Part print with two shaded views. Sizes in mm from the minimum x, y, z corner. Coordinates: 2 decimals unless noted, no trailing zeros. Loops run counter-clockwise (first coordinate to the right, second up) from the corner with the lowest first, then second, coordinate; pieces in that order, holes last.
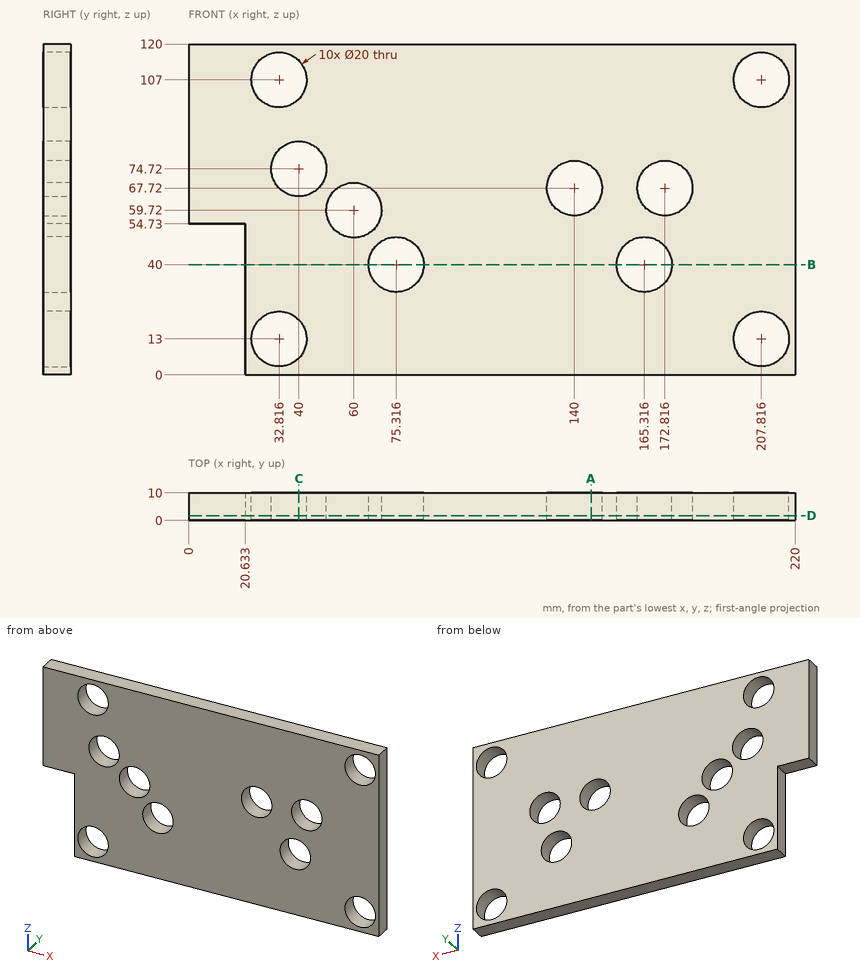
Q1. Drill centre lines: line 1 (X direction, y = 4.75, z = 13); line 2 (X direction, y = 5.5, z = 40); line 3 (X direction, y = 2.5, z = 67.72) (1 decimal). Where is each one in solid material? Low to high.
Answers:
line 1: x = 20.63 to 22.82, 42.82 to 197.82, 217.82 to 220
line 2: x = 20.63 to 65.32, 85.32 to 155.32, 175.32 to 220
line 3: x = 0 to 32.9, 47.1 to 54, 66 to 130, 150 to 162.8, 182.8 to 220
Q2. Flat gauge pins, fed straight in: P1, Ø23, axis at x = 207.82, z = 107, coming from the +Y side; P2, Ø5, axis at y = 3.5, z = 22.5, coming from the -X side. Where does each tip first touch, or does it go through?
Answers:
P1: stops at y = 10
P2: stops at x = 20.63
Q3. Slice it at C-C (x = 40). List the corners of the cut face in (y, z), and give its area (3 significant figures).
Answers:
outline: (0, 0) - (10, 0) - (10, 6.04) - (0, 6.04) - close; (0, 19.96) - (10, 19.96) - (10, 64.72) - (0, 64.72) - close; (0, 84.72) - (10, 84.72) - (10, 100.04) - (0, 100.04) - close; (0, 113.96) - (10, 113.96) - (10, 120) - (0, 120) - close
area: 722 mm2
Q4. Slice it at A-A (x = 146). List the corners of the cut face in (y, z), and give its area (3 significant figures).
Answers:
outline: (0, 0) - (10, 0) - (10, 59.72) - (0, 59.72) - close; (0, 75.72) - (10, 75.72) - (10, 120) - (0, 120) - close
area: 1,040 mm2
Q5. Slice it at B-B (z = 40). List the corners of the cut face in (x, y), and give its area (3 significant figures).
Answers:
outline: (20.63, 0) - (65.32, 0) - (65.32, 10) - (20.63, 10) - close; (85.32, 0) - (155.32, 0) - (155.32, 10) - (85.32, 10) - close; (175.32, 0) - (220, 0) - (220, 10) - (175.32, 10) - close
area: 1,590 mm2
Q6. Slice it at D-D (y = 1.75). Count the separate pieces of the cut face and the enclosed holes in it, and give its area (3 significant figures).
Answers:
separate pieces: 1
enclosed holes: 10
area: 22,100 mm2
